Verification items for this drawing (mm, ordinates from the low corner). Round coordinates to 2 decimals unless told otherwise and drop trailing zeros. Order: outer loops, then holes, each group sorted by start corner. A loop starts at its lowest first (then second) coordinate and runs counter-clockwise, first axis right, second up. Notation, with made-up numbers: (71.5, 1.25) - (86.5, 1.25) arc R25 cw to (86.5, 21.25) - close; hole circle Ø2 at (79.5, 56.25). An arc over 180 degrees is marked (long way). Use a Markdown table: item, result. Add a question column.
(1) Section check A-A on z = 195. Record the boundary of the cut face in (x, y) (3 decimals).
(2) Thickness scan on line 1 along X through (y, z) = (3.75, 10); line 2 along Z through (x, y) = (195, 1.5) (3 decimals). Record the ranges inside material, lowest first. Write a range as [from, to].
(3) Section check B-B on x = 105. Record the boundary of the cut face in (y, z) (3 decimals).
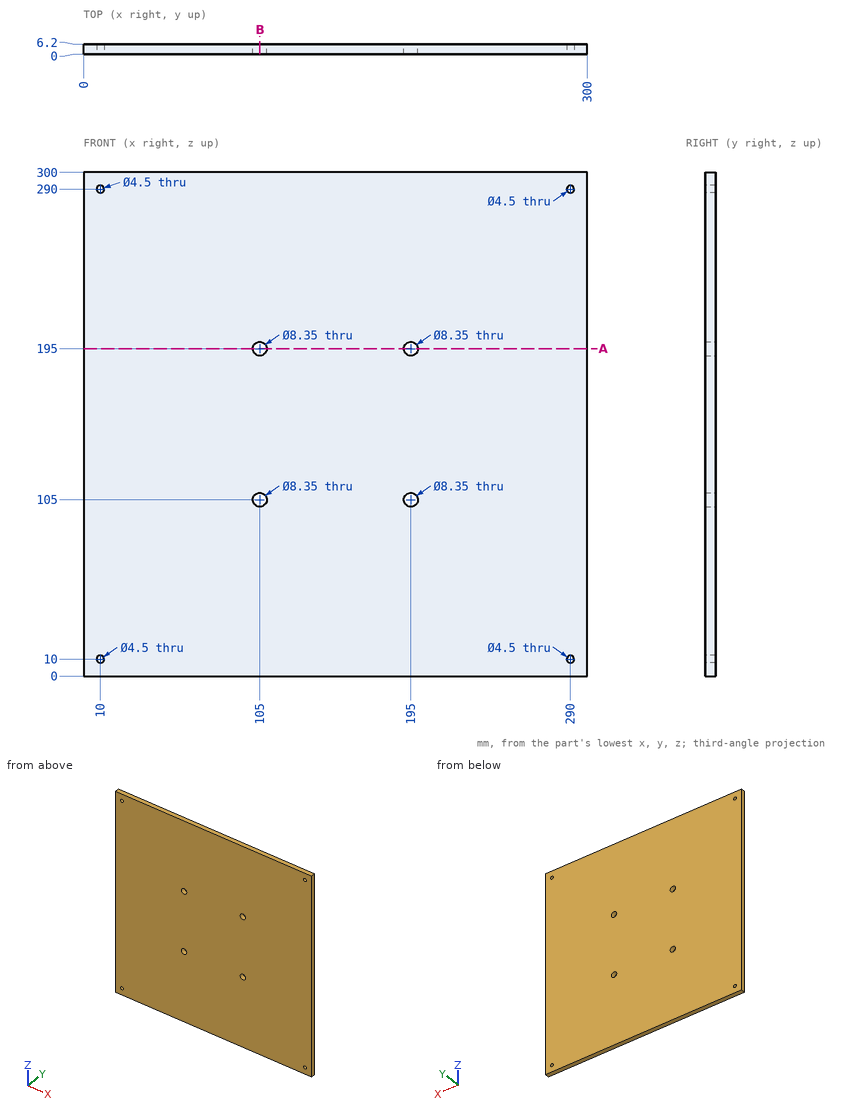
Check sheet entries:
| question | item | result |
|---|---|---|
| 1 | outline | (0, 0) - (100.825, 0) - (100.825, 6.2) - (0, 6.2) - close; (109.175, 0) - (190.825, 0) - (190.825, 6.2) - (109.175, 6.2) - close; (199.175, 0) - (300, 0) - (300, 6.2) - (199.175, 6.2) - close |
| 2 | line 1 | x = [0, 7.75], [12.25, 287.75], [292.25, 300] |
| 2 | line 2 | z = [0, 100.825], [109.175, 190.825], [199.175, 300] |
| 3 | outline | (0, 0) - (6.2, 0) - (6.2, 100.825) - (0, 100.825) - close; (0, 109.175) - (6.2, 109.175) - (6.2, 190.825) - (0, 190.825) - close; (0, 199.175) - (6.2, 199.175) - (6.2, 300) - (0, 300) - close |
